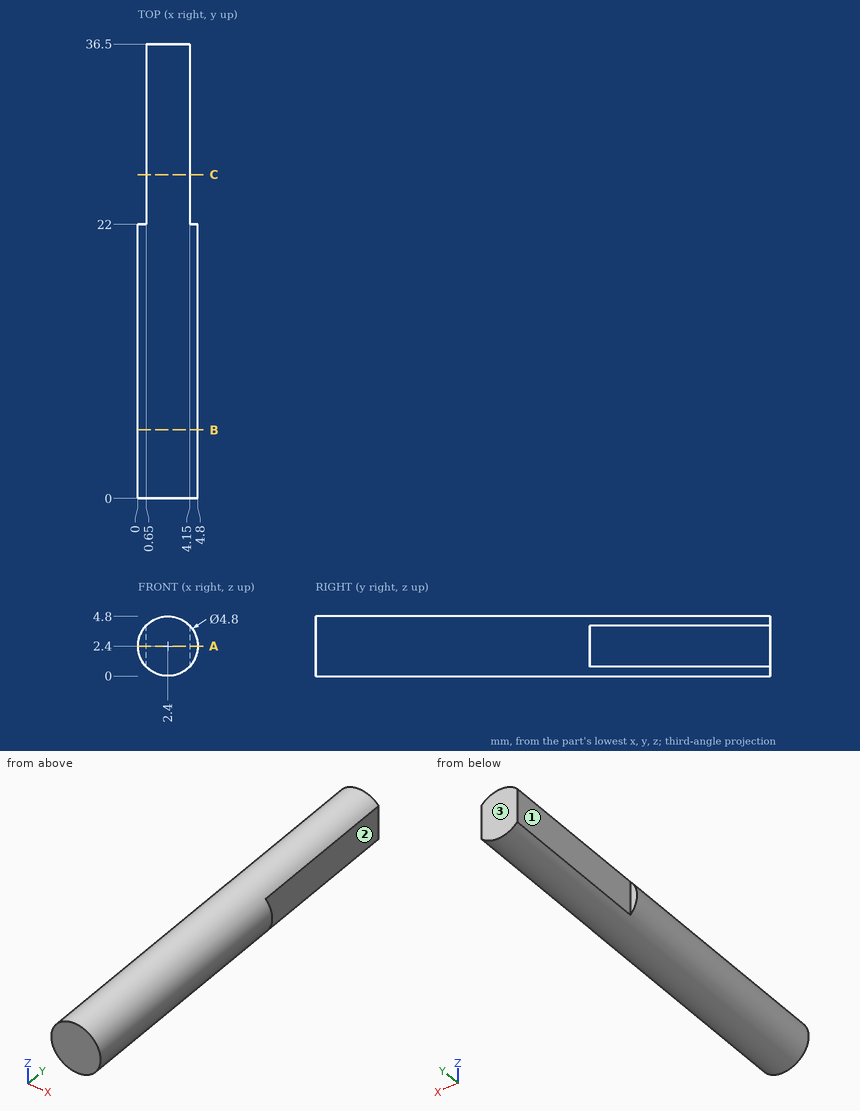
Here's the drawing with two shaded views (mm, measured from the low corner). I have some questions. A direction names the side the tool comes from. Coordinates: 2 decimals unless noted, no trailing zeros. Write each loop counter-clockwise with the first axis right and the second up, starting at its lowest first coordinate (ties: lowest second). Pieces come first, ordered by that corner, then holes. Notation, with made-up numbers: (72.25, 43.5) -> (131.25, 43.5) arc R28 cw to (131.25, 72.5) -> close; hole circle Ø11 at (29, 53.5). An arc over 180 degrees is marked (long way). One line per question, with ' | ' between items. Start each with the question number.
1. If we section it at C-C (y = 26): Please give me the cut outline in (x, z).
2. If we section it at A-A (z = 2.4): Please give me the cut outline in (x, y).
3. Will this pin go through, and if not, where does the flat tip stop? P1, Ø1, axis at y = 29, z = 3, coming from the -X side.
4. For the marked faces 1, 2 and 3, which set-ups out of +Z, -Z, +X, -X, +Y, -Y let a thin tool reach every point of the face, with its end or its side?
5. If we section it at B-B (y = 5.5): Please give me the cut outline in (x, z).
6. Please list where these lines run through material, in increasing order: line 1 along X through (y, z) = (29, 1.3); line 2 along X through (y, z) = (21.5, 2.55).
Return value:
1) outline: (0.65, 0.76) arc R2.4 ccw to (4.15, 0.76) -> (4.15, 4.04) arc R2.4 ccw to (0.65, 4.04) -> close
2) outline: (0, 0) -> (4.8, 0) -> (4.8, 22) -> (4.15, 22) -> (4.15, 36.5) -> (0.65, 36.5) -> (0.65, 22) -> (0, 22) -> close
3) P1: stops at x = 0.65
4) face 1: +Z, -Z, -X, +Y | face 2: +Z, -Z, +X, +Y | face 3: +Z, -Z, +X, -X, +Y
5) outline: circle Ø4.8 at (2.4, 2.4)
6) line 1: x = 0.65 to 4.15 | line 2: x = 0 to 4.8
